The listing builds one solid part. Answer for the finished solid, in the listing's coordinates (mm). Face numbers are marked on the shaded views. Round coordinates to 2 decimals unless told otherwise and drop trailing zeros. Write each loop counter-clockwise with the first axis right and the second up, starting at its lowest first coordinate (ties: lowest second). Pieces come first, ordered by that corner, then holes. Notation, with made-up numbers: (9, 65.25) - (38, 65.25) arc R33 ccw to (38, 93.25) - close; hole circle Ø6 at (55.25, -31). An arc over 180 degrees is marked (long way). Use a Markdown table: item, result. Add a question column.
1) Determine the mould class of the marked faces 1, 2, 3 and 4 for opening direction Y: +Y half, -Y half, draft (parallel to the pull), parting line (faces both ways), or undercut.
2) A cutting plane is placed at A-A (x = 8.25). Give the vertices of the cut face in (y, z).
3) Find the intervals of material crossed by probe 1 along Y at (x, z) = (7, 6.75); probe 2 along Z at (x, y) = (3, -1.65); probe 3 along X at (y, z) = (-2.3, 11.25), in increasing order. Write a range as from..to.
4) A cutting plane is placed at C-C (y = -1.85). Give the vertices of the cut face in (x, z), then the cut area to 3 significant figures.
5) A cutting plane is placed at B-B (z = 1.75). Give the vertices of the cut face in (x, y), then the cut area to 3 significant figures.
```python
from build123d import *

# Parameters (mm, degrees)
F0_W     = 10
F0_H     = 12.5
F1_DEPTH = 3
F2_W     = 1.9
F2_H     = 12
F3_DEPTH = 8


# Not quite as in the source:
# - a feature names something its author has since deleted; it is built from what else it names


with BuildPart() as f1:
    # F0 (on Front) → F1 (new body)
    with BuildSketch(Plane.XZ):
        with Locations((5, 6.25)):
            Rectangle(F0_W, F0_H)
    extrude(amount=F1_DEPTH)

    # F2 (on face) → F3 (cut)
    with BuildSketch(Plane.YZ.offset(10)):
        with Locations((-1.4556478869, 6.5)):
            Rectangle(F2_W, F2_H)
    extrude(amount=-F3_DEPTH, mode=Mode.SUBTRACT)


solid = f1.part
```
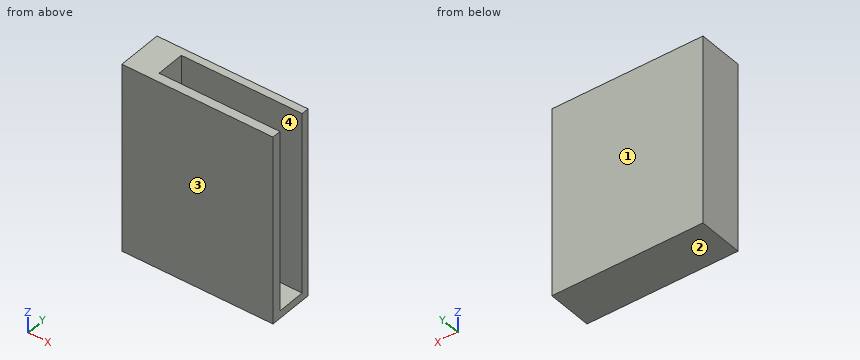
Entries:
| question | item | result |
|---|---|---|
| 1 | face 1 | +Y half |
| 1 | face 2 | draft |
| 1 | face 3 | -Y half |
| 1 | face 4 | undercut |
| 2 | outline | (-3, 0) - (0, 0) - (0, 12.5) - (-0.51, 12.5) - (-0.51, 0.5) - (-2.41, 0.5) - (-2.41, 12.5) - (-3, 12.5) - close |
| 3 | probe 1 | y = -3..-2.41, -0.51..0 |
| 3 | probe 2 | z = 0..0.5 |
| 3 | probe 3 | x = 0..2 |
| 4 | outline | (0, 0) - (10, 0) - (10, 0.5) - (2, 0.5) - (2, 12.5) - (0, 12.5) - close |
| 4 | area | 29.0 mm² |
| 5 | outline | (0, -3) - (10, -3) - (10, -2.41) - (2, -2.41) - (2, -0.51) - (10, -0.51) - (10, 0) - (0, 0) - close |
| 5 | area | 14.8 mm² |
